Source: CAD feature listing. Evaluate the final solid. Frame: model axes, mm. Coordinates: 2 decimals unless noted, no trailing zeros. Loops run counter-clockwise (first coordinate to the right, second up) from the corner with the lowest first, then second, coordinate; pieces in that order, holes last.
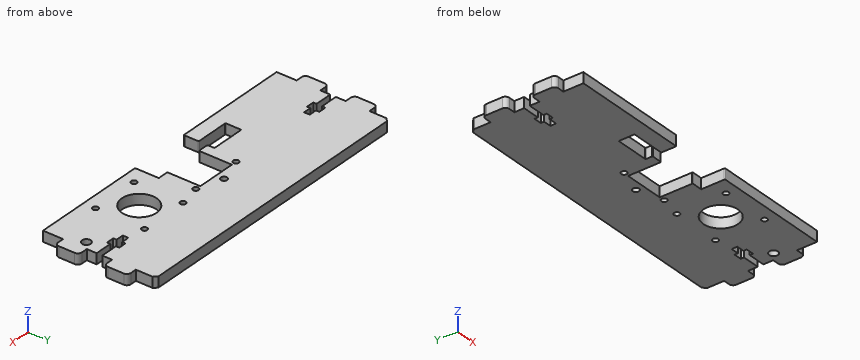
from build123d import *

# Parameters (mm, degrees)
MODEL_R             = 1.7526
MODEL_R_2           = 10.975
MODEL_R_3           = 2
MODEL_R_4           = 2.75
MODEL_R_5           = 1.775
BOSS_EXTRUDE1_DEPTH = 6.6


with BuildPart() as part:
    # Model → Boss-Extrude1 (new body)
    with BuildSketch(Plane.XY):
        with BuildLine():
            Line((0, 0), (74.150001665, 0))
            ThreePointArc((74.150001665, 0), (74.503555056, 0.146446609), (74.650001665, 0.5))
            Line((74.650001665, 0.5), (74.650001665, 8.9613))
            ThreePointArc((74.650001665, 8.9613), (74.503555056, 9.314853391), (74.150001665, 9.4613))
            Line((74.150001665, 9.4613), (53.610001665, 9.4613))
            ThreePointArc((53.610001665, 9.4613), (53.256448274, 9.607746609), (53.110001665, 9.9613))
            Line((53.110001665, 9.9613), (53.110001665, 18.9557))
            ThreePointArc((53.110001665, 18.9557), (53.256448274, 19.309253391), (53.610001665, 19.4557))
            Line((53.610001665, 19.4557), (74.150001665, 19.4557))
            ThreePointArc((74.150001665, 19.4557), (74.503555056, 19.309253391), (74.650001665, 18.9557))
            Line((74.650001665, 18.9557), (74.650001665, 15.5))
            ThreePointArc((74.650001665, 15.5), (74.796448274, 15.146446609), (75.150001665, 15))
            Line((75.150001665, 15), (81.010001665, 15))
            ThreePointArc((81.010001665, 15), (81.363555056, 15.146446609), (81.510001665, 15.5))
            Line((81.510001665, 15.5), (81.510001665, 35.87480678))
            Line((81.510001665, 35.87480678), (106.910001664, 35.87480678))
            Line((106.910001664, 35.87480678), (106.910001664, 15.5))
            ThreePointArc((106.910001664, 15.5), (107.056448274, 15.146446609), (107.410001664, 15))
            Line((107.410001664, 15), (113.770001664, 15))
            Line((113.770001664, 15), (113.770001664, 0.5))
            ThreePointArc((113.770001664, 0.5), (113.916448274, 0.146446609), (114.270001664, 0))
            Line((114.270001664, 0), (187.8, 0))
            Line((187.8, 0), (187.8, 12.7))
            Line((187.8, 12.7), (191.8, 12.7))
            ThreePointArc((191.8, 12.7), (193.567766953, 13.432233047), (194.3, 15.2))
            Line((194.3, 15.2), (194.3, 25.2))
            ThreePointArc((194.3, 25.2), (193.567766953, 26.967766953), (191.8, 27.7))
            Line((191.8, 27.7), (187.8, 27.7))
            Line((187.8, 27.7), (187.8, 33.935))
            Line((187.8, 33.935), (176.8, 33.935))
            Line((176.8, 33.935), (176.8, 31.85))
            Line((176.8, 31.85), (171.8, 31.85))
            Line((171.8, 31.85), (171.8, 33.935))
            Line((171.8, 33.935), (166.8, 33.935))
            Line((166.8, 33.935), (166.8, 37.485))
            Line((166.8, 37.485), (171.8, 37.485))
            Line((171.8, 37.485), (171.8, 39.57))
            Line((171.8, 39.57), (176.8, 39.57))
            Line((176.8, 39.57), (176.8, 37.485))
            Line((176.8, 37.485), (187.8, 37.485))
            Line((187.8, 37.485), (187.8, 43.72))
            Line((187.8, 43.72), (191.8, 43.72))
            ThreePointArc((191.8, 43.72), (193.567766953, 44.452233047), (194.3, 46.22))
            Line((194.3, 46.22), (194.3, 56.22))
            ThreePointArc((194.3, 56.22), (193.567766953, 57.987766953), (191.8, 58.72))
            Line((191.8, 58.72), (187.8, 58.72))
            Line((187.8, 58.72), (187.8, 69.42))
            Line((187.8, 69.42), (185.8, 71.42))
            Line((185.8, 71.42), (2, 71.42))
            Line((2, 71.42), (0, 69.42))
            Line((0, 69.42), (0, 58.72))
            Line((0, 58.72), (-4, 58.72))
            ThreePointArc((-4, 58.72), (-5.767766953, 57.987766953), (-6.5, 56.22))
            Line((-6.5, 56.22), (-6.5, 46.22))
            ThreePointArc((-6.5, 46.22), (-5.767766953, 44.452233047), (-4, 43.72))
            Line((-4, 43.72), (0, 43.72))
            Line((0, 43.72), (0, 37.485))
            Line((0, 37.485), (11, 37.485))
            Line((11, 37.485), (11, 39.57))
            Line((11, 39.57), (16, 39.57))
            Line((16, 39.57), (16, 37.485))
            Line((16, 37.485), (21, 37.485))
            Line((21, 37.485), (21, 33.935))
            Line((21, 33.935), (16, 33.935))
            Line((16, 33.935), (16, 31.85))
            Line((16, 31.85), (11, 31.85))
            Line((11, 31.85), (11, 33.935))
            Line((11, 33.935), (0, 33.935))
            Line((0, 33.935), (0, 27.7))
            Line((0, 27.7), (-4, 27.7))
            ThreePointArc((-4, 27.7), (-5.767766953, 26.967766953), (-6.5, 25.2))
            Line((-6.5, 25.2), (-6.5, 15.2))
            ThreePointArc((-6.5, 15.2), (-5.767766953, 13.432233047), (-4, 12.7))
            Line((-4, 12.7), (0, 12.7))
            Line((0, 12.7), (0, 0))
        make_face()
        with Locations((155.352001664, 38.674806781)):
            Circle(MODEL_R, mode=Mode.SUBTRACT)
        with Locations((155.352001664, 7.674806781)):
            Circle(MODEL_R, mode=Mode.SUBTRACT)
        with Locations((124.352001664, 38.674806781)):
            Circle(MODEL_R, mode=Mode.SUBTRACT)
        with Locations((124.352001664, 7.674806781)):
            Circle(MODEL_R, mode=Mode.SUBTRACT)
        with Locations((139.852001664, 23.174806781)):
            Circle(MODEL_R_2, mode=Mode.SUBTRACT)
        with Locations((94.210001665, 40.87480678)):
            Circle(MODEL_R_3, mode=Mode.SUBTRACT)
        with Locations((182.8, 23.5)):
            Circle(MODEL_R_4, mode=Mode.SUBTRACT)
        with Locations((110.340001664, 35.71)):
            Circle(MODEL_R_5, mode=Mode.SUBTRACT)
        with Locations((78.080001665, 35.71)):
            Circle(MODEL_R_5, mode=Mode.SUBTRACT)
    extrude(amount=BOSS_EXTRUDE1_DEPTH)


solid = part.part
Q1. Contact query for flat-ended pins moving along their axis: pin 1 Ø3 at (x, z) = (-2, 4.5) entering from -Y; pin 2 Ø3.5 at (x, z) = (89.5, 4.5) entering from -Y; pin 3 Ø1.2 at (x, z) = (189.5, 3) entering from +Y. Output: stop coordinate, or through.
Q2. Section B-B, the plane x = 100.5. Return the cut outline in (y, z).
Q3. Section C-C, the plane z = 4.5. Count the separate pieces of the cut face and the enclosed holes in it, plus the area to 3 significant figures.
Q4. Section A-A, the plane x = 182.8. Return the cut outline in (y, z) (3 decimals), plus the area to 3 significant figures.
Q5. Line query: line 1 along Y through (x, z) = (10, 5.75) (3 decimals); line 2 along X through (y, z) = (18, 3.5); line 3 along X through (y, z) = (10, 1.75). Output: solid intervals per line, ascending.
Derived:
1. pin 1: stops at y = 12.7
1. pin 2: stops at y = 35.87
1. pin 3: stops at y = 58.72
2. outline: (35.87, 0) - (71.42, 0) - (71.42, 6.6) - (35.87, 6.6) - close
3. separate pieces: 1
3. enclosed holes: 9
3. area: 11,800 mm2
4. outline: (0, 0) - (20.75, 0) - (20.75, 6.6) - (0, 6.6) - close; (26.25, 0) - (33.935, 0) - (33.935, 6.6) - (26.25, 6.6) - close; (37.485, 0) - (71.42, 0) - (71.42, 6.6) - (37.485, 6.6) - close
4. area: 412 mm2
5. line 1: y = 0 to 33.935, 37.485 to 71.42
5. line 2: x = -6.5 to 53.11, 74.65 to 81.51, 106.91 to 130.17, 149.53 to 194.3
5. line 3: x = 0 to 53.11, 113.77 to 187.8
